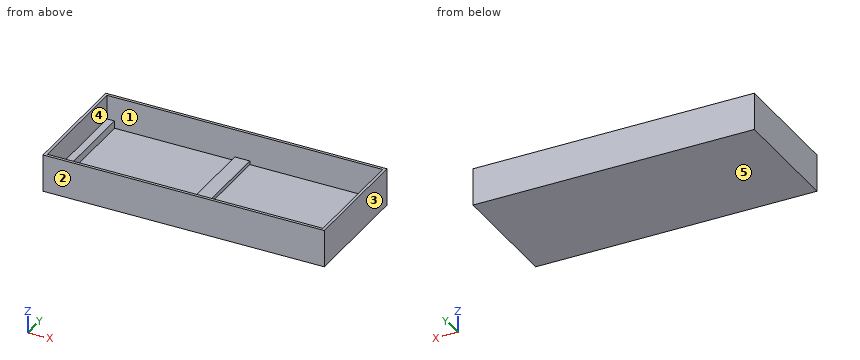
```python
from build123d import *

# Parameters (mm, degrees)
F0_W     = 1905
F0_H     = 254
F1_DEPTH = 406.4
F2_W     = 1866.9
F2_H     = 774.7
F3_DEPTH = 215.9
F4_W     = 50.8
F4_H     = 774.7
F5_DEPTH = 50.8
F6_W     = 101.6
F6_H     = 774.7
F7_DEPTH = 25.4


with BuildPart() as f1:
    # F0 (on Front) → F1 (new body, symmetric)
    with BuildSketch(Plane.XZ):
        with Locations((17.253051, 1.14385)):
            Rectangle(F0_W, F0_H)
    extrude(amount=F1_DEPTH, both=True)

    # F2 (on face) → F3 (cut)
    with BuildSketch(Plane.XY.offset(128.14385)):
        with Locations((17.253051, 0)):
            Rectangle(F2_W, F2_H)
    extrude(amount=-F3_DEPTH, mode=Mode.SUBTRACT)

    # F4 (on face) → F5 (join)
    with BuildSketch(Plane.XY.offset(-87.75615)):
        with Locations((-890.796949, 0)):
            Rectangle(F4_W, F4_H)
        with Locations((925.303051, 0)):
            Rectangle(F4_W, F4_H)
    extrude(amount=F5_DEPTH)

    # F6 (on face) → F7 (join)
    with BuildSketch(Plane.XY.offset(-87.75615)):
        Rectangle(F6_W, F6_H)
    extrude(amount=F7_DEPTH)


solid = f1.part
```
The listing builds one solid part. Answer for the finished solid, in the listing's coordinates (mm). Face numbers are marked on the shaded views. A direction names the side the tool comes from. Give positions to 0.01 mm unless a question says otherwise; leave off trailing zeros. Order: outer loops, then holes, each group sorted by start corner. A loop starts at its lowest first (then second) coordinate and runs counter-clockwise, first axis right, second up. Notation, with made-up numbers: (-12.75, 33.5) -> (4.25, 33.5) arc R30 ccw to (4.25, 62.5) -> close; hole circle Ø3 at (-24.75, 83). An arc over 180 degrees is marked (long way). One line per item, written item: value.
1) Determine the mould class of the marked faces 3, 4 and 5 for opening direction X: pulls with the +X half, pulls with the -X half, needs draft (parallel to the pull), parting line crosses it, or undercut.
Reported:
face 3: pulls with the +X half
face 4: undercut
face 5: needs draft
2) Flat-ended cylindrical pins translate along their axes: P1, Ø15, axis at x = 932.5, y = 93, coming from the +Z side; P2, Ø1, axis at x = 287, y = -262.5, coming from the +Z side. Find the tip coordinate at first contact, or state that the pin passes through.
Reported:
P1: stops at z = -36.96
P2: stops at z = -87.76
3) Find section A-A, the plane z = 8.5. Determine the outline of the cut face in (x, y).
Reported:
outline: (-935.25, -406.4) -> (969.75, -406.4) -> (969.75, 406.4) -> (-935.25, 406.4) -> close; hole (-916.2, -387.35) -> (950.7, -387.35) -> (950.7, 387.35) -> (-916.2, 387.35) -> close
4) Find the intervals of material crossed by line 1 (X direction, y = 326, z = -63); line 2 (Y direction, x = -22, z = -48); line 3 (X direction, y = -297, z = -50), in increasing order.
Reported:
line 1: x = -935.25 to -865.4, -50.8 to 50.8, 899.9 to 969.75
line 2: y = -406.4 to -387.35, 387.35 to 406.4
line 3: x = -935.25 to -865.4, 899.9 to 969.75
5) Find section C-C, the plane x = 387. Determine the outline of the cut face in (y, z), plus the area to 3 significant figures.
Reported:
outline: (-406.4, -125.86) -> (406.4, -125.86) -> (406.4, 128.14) -> (387.35, 128.14) -> (387.35, -87.76) -> (-387.35, -87.76) -> (-387.35, 128.14) -> (-406.4, 128.14) -> close
area: 39,200 mm^2
6) A tool of negligible diameter and unlimited length cuts with its end or side. For the marked faces 1 and 2, from which of +Z, -Z, +X, -X, +Y, -Y can it reach the whole face along a straight path? Write none if from no direction.
Reported:
face 1: +Z
face 2: +Z, -Z, +X, -X, -Y
7) Find section B-B, the plane y = 28.5. Determine the outline of the cut face in (x, z).
Reported:
outline: (-935.25, -125.86) -> (969.75, -125.86) -> (969.75, 128.14) -> (950.7, 128.14) -> (950.7, -36.96) -> (899.9, -36.96) -> (899.9, -87.76) -> (50.8, -87.76) -> (50.8, -62.36) -> (-50.8, -62.36) -> (-50.8, -87.76) -> (-865.4, -87.76) -> (-865.4, -36.96) -> (-916.2, -36.96) -> (-916.2, 128.14) -> (-935.25, 128.14) -> close
